Verification items for this drawing (mm, ordinates from the low corner). Round coordinates to 2 decimals unless told otherwise and drop trailing zeros. Order: outer loops, then holes, each group sorted by start corner. A loop starts at its lowest first (then second) coordinate and runs counter-clockwise, first axis right, second up. Notation, with made-up numbers: (51, 2) -> (63, 2) arc R21 cw to (63, 18) -> close; hole circle Ø7 at (10.25, -17.5). An arc over 180 degrees is marked (long way). Put each result on its own line as item: value.
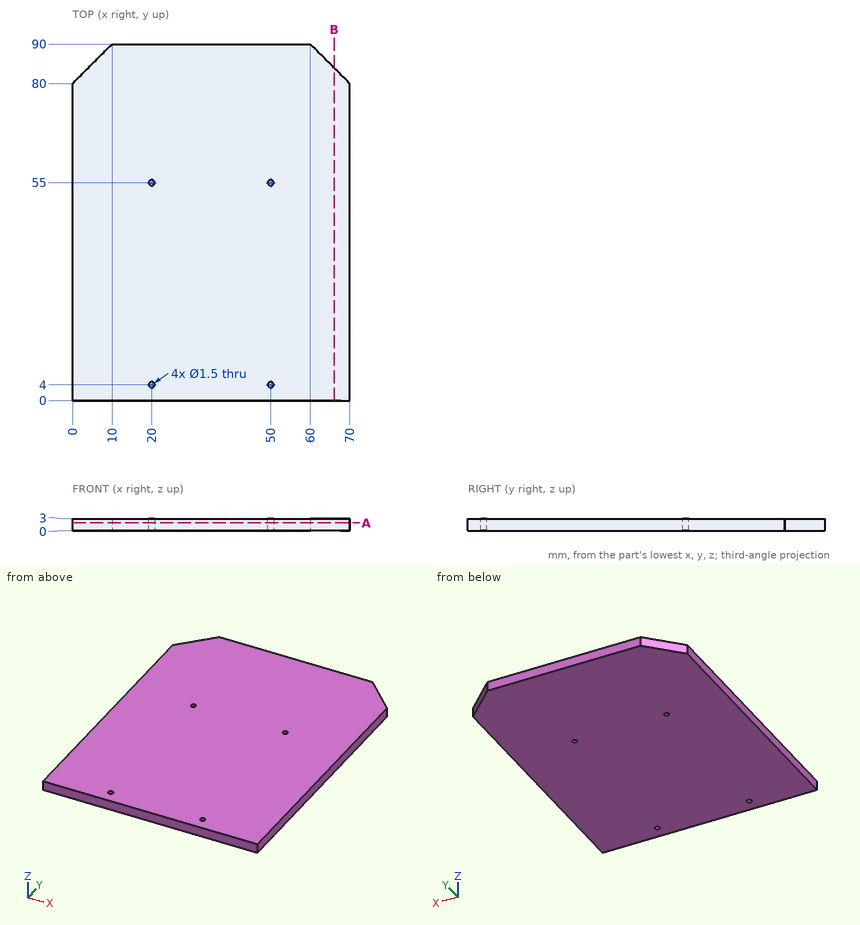
Item 1: Section check B-B on x = 66. Record the boundary of the cut face in (y, z).
Check sheet entries:
outline: (0, 0) -> (84, 0) -> (84, 3) -> (0, 3) -> close
Item 2: Section check A-A on z = 1.9. Record the boundary of the cut face in (x, y).
Check sheet entries:
outline: (0, 0) -> (70, 0) -> (70, 80) -> (60, 90) -> (10, 90) -> (0, 80) -> close; hole circle Ø1.5 at (20, 4); hole circle Ø1.5 at (20, 55); hole circle Ø1.5 at (50, 4); hole circle Ø1.5 at (50, 55)
Item 3: Material ranges on L1, parallel to Y at x = 20, z = 2.45; L2, parallel to X at y = 4.5, z = 1.65; L3, parallel to Y at x = 62.5, z = 1.6, recorded low to high. Write a range as [from, to].
Check sheet entries:
L1: y = [0, 3.25], [4.75, 54.25], [55.75, 90]
L2: x = [0, 19.44], [20.56, 49.44], [50.56, 70]
L3: y = [0, 87.5]
